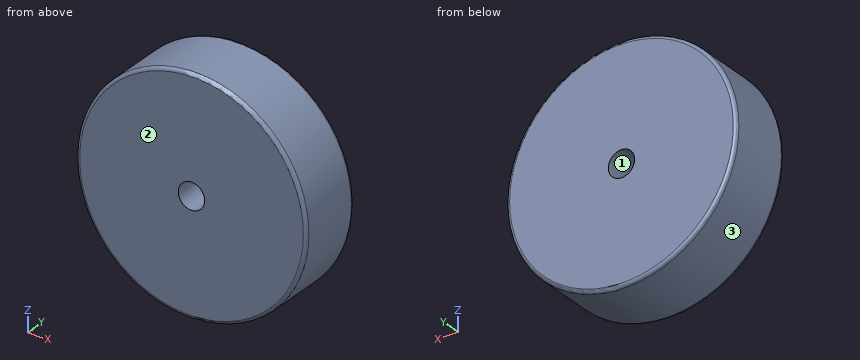
from build123d import *

# Parameters (mm, degrees)
F0_R     = 17.4625
F1_DEPTH = 10.16
F2_R     = 2
F3_DEPTH = 25.4
F4_R     = 0.5


with BuildPart() as f1:
    # F0 (on Front) → F1 (new body)
    with BuildSketch(Plane.XZ):
        Circle(F0_R)
    extrude(amount=F1_DEPTH)

    # F2 (on face) → F3 (cut)
    with BuildSketch(Plane.XZ.offset(10.16)):
        Circle(F2_R)
    extrude(amount=-F3_DEPTH, mode=Mode.SUBTRACT)

    # F4
    f4_edges = [f1.edges().sort_by_distance(p)[0] for p in [
        (-17.4625, -10.16, 0),
        (-17.4625, 0, 0),
    ]]
    fillet(f4_edges, radius=F4_R)


solid = f1.part
CAD build for the part. Positions are in the model's coordinates, mm. Face numbers are marked on the shaded views. Round coordinates to 2 decimals unless told otherwise and drop trailing zeros. Loops run counter-clockwise (first coordinate to the right, second up) from the corner with the lowest first, then second, coordinate; pieces in that order, holes last.
(1) Cut at B-B (z = 0). Give the cut face in (x, y), plus the area to 3 significant figures.
(2) Cut at C-C (y = -6.5). Give the cut face in (x, z) (1 decimal), plus the area to 3 significant figures.
(3) Cut at A-A (x = 0). Give the cut face in (y, z), plus the area to 3 significant figures.
(4) Wall check: line 1 along Z through (x, y) = (0, -4.5); line 2 along Z through (x, y) = (-10, -6.25); line 3 along Z through (x, y) = (-12, -3.5). Give the ranges that are in metal, low to high.
(5) Two-plate mould, pull along Z, no slides. Class the marked faces 1, 2 and 3: +Z half, -Z half, draft (parallel to the pull), parting line (faces both ways), or undercut.
(6) Drop flat-ended pins along their axis: pin 1 (5 mm diameter, centred on y = -1, z = -5.5, fed in from -X); pin 2 (1 mm diameter, centred on x = -4.5, y = -4.5, fed in from +Z); pin 3 (1.5 mm diameter, centred on y = -1.5, z = 10.5, fed in from -X). Give the stop position or say it passes through.
Findings below:
1. outline: (-17.46, -9.66) arc R0.5 ccw to (-16.96, -10.16) - (-2, -10.16) - (-2, 0) - (-16.96, 0) arc R0.5 ccw to (-17.46, -0.5) - close; (2, -10.16) - (16.96, -10.16) arc R0.5 ccw to (17.46, -9.66) - (17.46, -0.5) arc R0.5 ccw to (16.96, 0) - (2, 0) - close
1. area: 314 mm2
2. outline: circle Ø34.9 at (0, 0); hole circle Ø4 at (0, 0)
2. area: 945 mm2
3. outline: (-10.16, -16.96) arc R0.5 ccw to (-9.66, -17.46) - (-0.5, -17.46) arc R0.5 ccw to (0, -16.96) - (0, -2) - (-10.16, -2) - close; (-10.16, 2) - (0, 2) - (0, 16.96) arc R0.5 ccw to (-0.5, 17.46) - (-9.66, 17.46) arc R0.5 ccw to (-10.16, 16.96) - close
3. area: 314 mm2
4. line 1: z = -17.46 to -2, 2 to 17.46
4. line 2: z = -14.32 to 14.32
4. line 3: z = -12.69 to 12.69
5. face 1: undercut
5. face 2: draft
5. face 3: parting line
6. pin 1: stops at x = -17.2
6. pin 2: stops at z = 17
6. pin 3: stops at x = -14.49
